Geometry: final body of the model. Coordinates: model frame, mm. A direction names the side the tool comes from. Give positions to 0.01 mm unless a question says otherwise; leave off trailing zeros. Order: outer loops, then holes, each group sorted by start corner. A loop starts at its lowest first (then second) coordinate and runs counter-clockwise, first axis right, second up. Notation, with made-up numbers: (44.5, -24) -> (84.5, -24) arc R14 ccw to (84.5, 3) -> close; hole circle Ø8 at (68.5, -23.5). An arc over 180 degrees is marked (long way). One line per question, with ' | ' between items. Start each with the question number.
(1) Mould query, pull axis Y, two halves, no side actions, for faces 3 (the face through (4.57, -6.2, 1.38)), 4 (the face through (0, 6, -5)), 5 (the face through (2.691, 3.834, -12.174)). Classes: +Y half, -Y half, draft (parallel to the pull), parting line (faces both ways), or undercut.
(2) Ray query, L1, parallel to Y at x = 4, z = 0; L2, parallel to Z at x = 5, y = 0.5; L3, parallel to Z at x = 3.75, y = -4.5. Return the intervals inside material, ascending.
(3) Set-up query: faces 1 (the face through (1.27, -8, 9)), 2 (the face through (7.963, -6, -4)). Return all of +Z, -Z, +X, -X, +Y, -Y with unobstructed straight access to the full face (end or side cutting, diameter ignored); none if empty.
(4) First-contact query: pin 1 Ø1.5 at (x, z) = (5, 0.5) entering from +Y; pin 2 Ø1 at (y, z) = (7, -9) entering from -X; pin 3 Ø2 at (x, y) = (3, 2.5) entering from +Z. Flat tips, straight axial feed; report the tip coordinate or a pass-through.
(5) Section C-C (x = 2). Return loops of the section in (y, z), then the cut area to 3 significant figures.
(6) Section D-D (x = 7.25). Return loops of the section in (y, z).
```python
from build123d import *

# Parameters (mm, degrees)
SKETCH1_R           = 12.7635
SKETCH1_R_2         = 6.35
BOSS_EXTRUDE1_DEPTH = 7.9629
FILLET1_R           = 3.81
SKETCH2_R           = 12.7635
SKETCH2_R_2         = 11.802652822
CUT_EXTRUDE1_DEPTH  = 1.27
FILLET2_R           = 1.27


with BuildPart() as part:
    # Sketch1 → Boss-Extrude1 (new body)
    with BuildSketch(Plane(origin=(0, 0, 0), x_dir=(0, 0, -1), z_dir=(1, 0, 0))):
        Circle(SKETCH1_R)
        Circle(SKETCH1_R_2, mode=Mode.SUBTRACT)
    extrude(amount=BOSS_EXTRUDE1_DEPTH)

    # Fillet1
    fillet1_edges = [part.edges().sort_by_distance(p)[0] for p in [
        (7.9629, 0, 12.7635),
    ]]
    fillet(fillet1_edges, radius=FILLET1_R)

    # Sketch2 → Cut-Extrude1 (cut)
    with BuildSketch(Plane.ZY):
        Circle(SKETCH2_R)
        Circle(SKETCH2_R_2, mode=Mode.SUBTRACT)
    extrude(amount=-CUT_EXTRUDE1_DEPTH, mode=Mode.SUBTRACT)

    # Fillet2
    fillet2_edges = [part.edges().sort_by_distance(p)[0] for p in [
        (0, 0, -11.802652822),
        (0, 0, 6.35),
    ]]
    fillet(fillet2_edges, radius=FILLET2_R - 0.0001)  # a hair under: the kernel refuses the full size


solid = part.part
```
Response:
1) face 3: undercut | face 4: draft | face 5: parting line
2) L1: y = -12.76 to -6.35, 6.35 to 12.76 | L2: z = -12.66 to -6.33, 6.33 to 12.66 | L3: z = -11.94 to -4.48, 4.48 to 11.94
3) face 1: -X | face 2: +Z, -Z, +X, +Y, -Y
4) pin 1: stops at y = 12.76 | pin 2: stops at x = 0.05 | pin 3: stops at z = 12.68
5) outline: circle Ø25.53 at (0, 0); hole circle Ø12.7 at (0, 0) | area: 385 mm^2
6) outline: circle Ø22.35 at (0, 0); hole circle Ø12.7 at (0, 0)
